Input: dimensioned drawing with shaded views. Units: mm. Origin: part minimum x, y, z. Give positions to 0.01 mm unless a question says otherwise; leave off trailing zeros. Order: outer loops, then holes, each group sorted by start corner. A loop starts at its lowest first (then second) coordinate and runs counter-clockwise, first axis right, second up. Notation, with made-up numbers: (-36, 41) - (16, 41) arc R35 ccw to (16, 79) - close; hole circle Ø1 at (-13, 66). An arc over 180 degrees is marked (long way). Use a Markdown table: item, result.
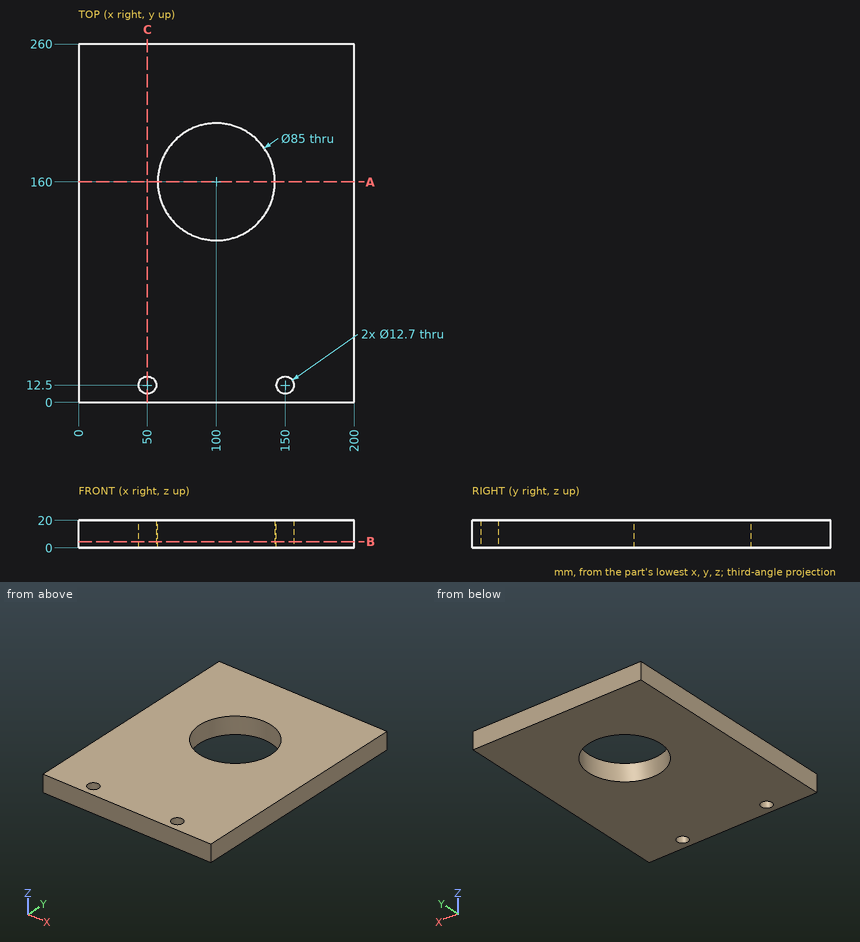
1. Section query B-B (z = 4.5). Return loops of the section in (x, y).
Response:
| item | result |
|---|---|
| outline | (0, 0) - (200, 0) - (200, 260) - (0, 260) - close; hole circle Ø12.7 at (50, 12.5); hole circle Ø85 at (100, 160); hole circle Ø12.7 at (150, 12.5) |
2. Material intervals for line 1 along Y through (x, z) = (150, 14.25); line 2 along Y through (x, z) = (100, 9.75); line 3 along X through (y, z) = (122, 8), sorted ascending.
Response:
| item | result |
|---|---|
| line 1 | y = 0 to 6.15, 18.85 to 260 |
| line 2 | y = 0 to 117.5, 202.5 to 260 |
| line 3 | x = 0 to 80.97, 119.03 to 200 |
3. Pin query (flat end, axial travel): pin 1 (10 mm diameter, centred on x = 50, y = 12.5, fed in from -Z). Return the tip coordinate at first contact, or that it passes through.
Response:
| item | result |
|---|---|
| pin 1 | passes through |
4. Section query C-C (x = 50). Return loops of the section in (y, z).
Response:
| item | result |
|---|---|
| outline | (0, 0) - (6.15, 0) - (6.15, 20) - (0, 20) - close; (18.85, 0) - (260, 0) - (260, 20) - (18.85, 20) - close |
5. Section query A-A (y = 160). Return loops of the section in (x, z), then the cut area to 3 significant figures.
Response:
| item | result |
|---|---|
| outline | (0, 0) - (57.5, 0) - (57.5, 20) - (0, 20) - close; (142.5, 0) - (200, 0) - (200, 20) - (142.5, 20) - close |
| area | 2,300 mm^2 |
